Build history of the part. All positions in model axes, mm. A direction names the side the tool comes from. Coordinates: 2 decimals unless noted, no trailing zeros. Write each loop counter-clockwise with the first axis right and the second up, starting at its lowest first coordinate (ties: lowest second). Pieces come first, ordered by that corner, then holes. Notation, with made-up numbers: (13.5, 23.5) -> (17.5, 23.5) arc R19 cw to (17.5, 49.5) -> close; hole circle Ø9 at (-6.5, -20.75). An arc over 180 degrees is marked (long way). Write each question's results on one line, items separated by ' | '. Start each with the question number.
Q1. Two-plate mould, pull along Z, no slides. Class faces 3 (the face through (0.413, -4.732, -2.461)), 4 (the face through (0.838, 3, 4)), 5 (the face through (0.051, 4, 0)): released by +Z, released by -Z, zero draft, split by the parting line, or undercut.
Q2. Drop a flat-ended pin along its axis: pin 1 Ø4 at (y, z) = (3.5, 3) entering from -X. Give the stop position or say it passes through.
Q3. Saw through at C-C on x = 0.5. Give the cut face in (y, z) (3 decimals).
Q4. Drill centre lines: line 1 (Y direction, x = 0.9, z = 0) (1 decimal); line 2 (X direction, y = 4.75, z = -0.75); line 3 (Y direction, x = 0.55, z = 0) (3 decimals). Where is each one in solid material? Low to high.
Q5. Tool access for faces 1 (the face through (1.98, -2.9, 3.78)), 2 (the face through (0, 4.4, 1.2)): list every direction of +Z, -Z, +X, -X, +Y, -Y with a clear straight run to the whole face (end or side of a thin tool).
Q6. Saw through at D-D on y = 3.75. Give the cut face in (x, z).
from build123d import *

# Parameters (mm, degrees)
SKETCH1_R           = 5.334
BOSS_EXTRUDE1_DEPTH = 0.8382
SKETCH2_R           = 4.7625
BOSS_EXTRUDE2_DEPTH = 2.3114
SKETCH3_R           = 3.175
CUT_EXTRUDE1_DEPTH  = 9.174539263
SKETCH4_R           = 4.4069
SKETCH4_R_2         = 3.5433
CUT_EXTRUDE2_DEPTH  = 0.0508
CUT_EXTRUDE3_START  = -0.0508
SKETCH5_R           = 4.2545
SKETCH5_R_2         = 3.5433
CUT_EXTRUDE3_DEPTH  = 0.0508


with BuildPart() as part:
    # Sketch1 → Boss-Extrude1 (new body)
    with BuildSketch(Plane(origin=(0, 0, 0), x_dir=(0, 0, -1), z_dir=(1, 0, 0))):
        Circle(SKETCH1_R)
    extrude(amount=BOSS_EXTRUDE1_DEPTH)

    # Sketch2 → Boss-Extrude2 (add)
    with BuildSketch(Plane(origin=(0.8382, 0, 0), x_dir=(0, 0, -1), z_dir=(1, 0, 0))):
        Circle(SKETCH2_R)
    extrude(amount=BOSS_EXTRUDE2_DEPTH)

    # Sketch3 → Cut-Extrude1 (cut, through all)
    with BuildSketch(Plane(origin=(3.1496, 0, 0), x_dir=(0, 0, -1), z_dir=(1, 0, 0))):
        Circle(SKETCH3_R)
    extrude(amount=-CUT_EXTRUDE1_DEPTH, mode=Mode.SUBTRACT)

    # Sketch4 → Cut-Extrude2 (cut)
    with BuildSketch(Plane.ZY):
        Circle(SKETCH4_R)
        Circle(SKETCH4_R_2, mode=Mode.SUBTRACT)
    extrude(amount=-CUT_EXTRUDE2_DEPTH, mode=Mode.SUBTRACT)

    # Sketch5 → Cut-Extrude3 (cut)
    with BuildSketch(Plane(origin=(3.1496, 0, 0), x_dir=(0, 0, -1), z_dir=(1, 0, 0)).offset(CUT_EXTRUDE3_START)):
        Circle(SKETCH5_R)
        with Locations(Location((0, 0, 0), (0, 0, 180))):
            Circle(SKETCH5_R_2, mode=Mode.SUBTRACT)
    extrude(amount=CUT_EXTRUDE3_DEPTH, mode=Mode.SUBTRACT)


solid = part.part
Returned:
1) face 3: split by the parting line | face 4: zero draft | face 5: undercut
2) pin 1: stops at x = 0
3) outline: circle Ø10.668 at (0, 0); hole circle Ø6.35 at (0, 0)
4) line 1: y = -4.8 to -3.2, 3.2 to 4.8 | line 2: x = 0 to 0.84 | line 3: y = -5.334 to -3.175, 3.175 to 5.334
5) face 1: +X | face 2: +Z, -Z, -X, +Y, -Y
6) outline: (0, -3.79) -> (0.84, -3.79) -> (0.84, -2.94) -> (3.15, -2.94) -> (3.15, -2.01) -> (3.1, -2.01) -> (3.1, 2.01) -> (3.15, 2.01) -> (3.15, 2.94) -> (0.84, 2.94) -> (0.84, 3.79) -> (0, 3.79) -> (0, 2.31) -> (0.05, 2.31) -> (0.05, -2.31) -> (0, -2.31) -> close
